Input: part model. Units: mm. Frame: model coordinates. A direction names the side the tool comes from. Round coordinates to 2 decimals unless told otherwise and drop trailing zeros. Loops run counter-clockwise (first coordinate to the right, second up) from the corner with the lowest first, then second, coordinate; pieces in that order, holes last.
(1) Cut plane D-D, the plane z = 0. Output: boundary loops of the cut face in (x, y), and give its area (3 significant figures).
(2) Cut plane C-C, the plane y = -22.5. Output: boundary loops of the cut face in (x, z), and give its area (3 significant figures).
(3) Cut plane B-B, the plane z = 41.5. Output: boundary loops of the cut face in (x, y).
(4) Draft query along Z for faces 1 (the face through (-1, -35, 1)), 2 (the face through (61, -27, -51)), 3 (the face through (-1, -27, 62.5)), 4 (the face through (60, -27, -32)). Return one class per face: released by +Z, released by -Z, zero draft, split by the parting line, or undercut.
(5) Line query: line 1 (Z direction, x = 56, y = -31.5); line 2 (X direction, y = -16.75, z = 0); line 3 (X direction, y = -7, z = 0). Output: solid intervals per line, ascending.
(6) First-contact query: pin 1 Ø2 at (x, z) = (49.5, -30.5) entering from +Y; pin 2 Ø4 at (y, z) = (-16, 9) entering from +X; pin 3 Ø1 at (y, z) = (-28.5, -49) entering from +X. Flat tips, straight axial feed; report the tip coordinate or a pass-through.
(7) Cut plane A-A, the plane x = -38.5. Output: boundary loops of the cut face in (y, z), and give its area (4 significant figures).
(8) Access query for faces 5 (the face through (-12, -10, -12)), 6 (the face through (0.66, -4.93, -14.985)), 7 (the face through (-94.998, -27.395, 41.291)). Directions: +Z, -Z, +X, -X, +Y, -Y. A direction counts if a zero-diameter tool reaches every point of the face in a straight line with its end or side. Return the directions, or none.
from build123d import *

# Parameters (mm, degrees)
SKETCH1_R           = 20
SKETCH1_R_2         = 15
BOSS_EXTRUDE1_DEPTH = 5
SKETCH2_R           = 30
SKETCH2_R_2         = 15
BOSS_EXTRUDE2_DEPTH = 15
SKETCH3_R           = 27.5
CUT_EXTRUDE1_DEPTH  = 10
SKETCH4_W           = 200
SKETCH4_H           = 125
BOSS_EXTRUDE3_DEPTH = 15
FILLET1_R           = 15


with BuildPart() as part:
    # Sketch1 → Boss-Extrude1 (new body)
    with BuildSketch(Plane(origin=(0, 0, 0), x_dir=(1, 0, 0), z_dir=(0, 1, 0))):
        with Locations(Location((0, 0, 0), (0, 0, 270))):
            Circle(SKETCH1_R)
        with Locations(Location((0, 0, 0), (0, 0, 270))):
            Circle(SKETCH1_R_2, mode=Mode.SUBTRACT)
    extrude(amount=-BOSS_EXTRUDE1_DEPTH)

    # Sketch2 → Boss-Extrude2 (add)
    with BuildSketch(Plane.XZ.offset(5)):
        with Locations(Location((0, 0, 0), (0, 0, 270))):
            Circle(SKETCH2_R)
        with Locations(Location((0, 0, 0), (0, 0, 90))):
            Circle(SKETCH2_R_2, mode=Mode.SUBTRACT)
    extrude(amount=BOSS_EXTRUDE2_DEPTH)

    # Sketch3 → Cut-Extrude1 (cut)
    with BuildSketch(Plane.XZ.offset(20)):
        with Locations(Location((0, 0, 0), (0, 0, 270))):
            Circle(SKETCH3_R)
    extrude(amount=-CUT_EXTRUDE1_DEPTH, mode=Mode.SUBTRACT)

    # Sketch4 → Boss-Extrude3 (add)
    with BuildSketch(Plane.XZ.offset(20)):
        Rectangle(SKETCH4_W, SKETCH4_H)
        with BuildLine():
            Line((-85.5, 51), (-35.5, 51))
            ThreePointArc((-35.5, 51), (-26, 41.5), (-35.5, 32))
            Line((-35.5, 32), (-85.5, 32))
            ThreePointArc((-85.5, 32), (-95, 41.5), (-85.5, 51))
        make_face(mode=Mode.SUBTRACT)
        with BuildLine():
            Line((-85.5, -51), (-35.5, -51))
            ThreePointArc((-35.5, -51), (-26, -41.5), (-35.5, -32))
            Line((-35.5, -32), (-85.5, -32))
            ThreePointArc((-85.5, -32), (-95, -41.5), (-85.5, -51))
        make_face(mode=Mode.SUBTRACT)
        with BuildLine():
            Line((85.5, 51), (35.5, 51))
            ThreePointArc((35.5, 51), (26, 41.5), (35.5, 32))
            Line((35.5, 32), (85.5, 32))
            ThreePointArc((85.5, 32), (95, 41.5), (85.5, 51))
        make_face(mode=Mode.SUBTRACT)
        with BuildLine():
            Line((85.5, -51), (35.5, -51))
            ThreePointArc((35.5, -51), (26, -41.5), (35.5, -32))
            Line((35.5, -32), (85.5, -32))
            ThreePointArc((85.5, -32), (95, -41.5), (85.5, -51))
        make_face(mode=Mode.SUBTRACT)
    extrude(amount=BOSS_EXTRUDE3_DEPTH)

    # Fillet1
    fillet1_edges = [part.edges().sort_by_distance(p)[0] for p in [
        (100, -27.5, 62.5),
        (-100, -27.5, 62.5),
        (-100, -27.5, -62.5),
        (100, -27.5, -62.5),
    ]]
    fillet(fillet1_edges, radius=FILLET1_R)


solid = part.part
Reported:
1. outline: (-100, -35) - (100, -35) - (100, -20) - (30, -20) - (30, -5) - (20, -5) - (20, 0) - (15, 0) - (15, -10) - (27.5, -10) - (27.5, -20) - (-27.5, -20) - (-27.5, -10) - (-15, -10) - (-15, 0) - (-20, 0) - (-20, -5) - (-30, -5) - (-30, -20) - (-100, -20) - close
1. area: 3,250 mm2
2. outline: (-100, -47.5) arc R15 ccw to (-85, -62.5) - (85, -62.5) arc R15 ccw to (100, -47.5) - (100, 47.5) arc R15 ccw to (85, 62.5) - (-85, 62.5) arc R15 ccw to (-100, 47.5) - close; hole (-85.5, -51) - (-35.5, -51) arc R9.5 ccw to (-35.5, -32) - (-85.5, -32) arc R9.5 ccw to start; hole (-85.5, 32) - (-35.5, 32) arc R9.5 ccw to (-35.5, 51) - (-85.5, 51) arc R9.5 ccw to start; hole (35.5, -51) - (85.5, -51) arc R9.5 ccw to (85.5, -32) - (35.5, -32) arc R9.5 ccw to start; hole (35.5, 32) - (85.5, 32) arc R9.5 ccw to (85.5, 51) - (35.5, 51) arc R9.5 ccw to start
2. area: 19,900 mm2
3. outline: (-100, -35) - (-95, -35) - (-95, -20) - (-100, -20) - close; (-26, -35) - (26, -35) - (26, -20) - (-26, -20) - close; (95, -35) - (100, -35) - (100, -20) - (95, -20) - close
4. face 1: zero draft
4. face 2: undercut
4. face 3: released by +Z
4. face 4: undercut
5. line 1: z = -62.5 to -51, -32 to 32, 51 to 62.5
5. line 2: x = -30 to -27.5, 27.5 to 30
5. line 3: x = -30 to -15, 15 to 30
6. pin 1: stops at y = -20
6. pin 2: stops at x = 29.17
6. pin 3: stops at x = 99.97
7. outline: (-35, -62.5) - (-20, -62.5) - (-20, -51) - (-35, -51) - close; (-35, -32) - (-20, -32) - (-20, 32) - (-35, 32) - close; (-35, 51) - (-20, 51) - (-20, 62.5) - (-35, 62.5) - close
7. area: 1,305 mm2
8. face 5: none
8. face 6: +Y
8. face 7: +Y, -Y
